Build history of the part. All positions in model axes, mm. A direction names the side the tool comes from. Give positions to 0.01 mm unless a question says otherwise; leave off trailing zeros. Order: outer loops, then holes, each group sorted by start corner. A loop starts at its lowest first (then second) coordinate and runs counter-clockwise, first axis right, second up. Notation, with made-up numbers: M 67.25,18.25 L 75.25,18.25 A19 cw 75.25,34.25 Z; hole C 30.5,45 d7. An arc over 180 degrees is marked long. One line per item, written item: value. Start each with the question number.
from build123d import *

# Parameters (mm, degrees)
SKETCH4_R           = 72
BOSS_EXTRUDE3_DEPTH = 5
SKETCH3_R           = 4
CUT_EXTRUDE6_DEPTH  = 102.946064171
SKETCH2_R           = 1.6
CUT_EXTRUDE1_DEPTH  = 102.946064171
GOPRO_DEPTH         = 102.946064171


with BuildPart() as part:
    # Sketch4 → Boss-Extrude3 (new body)
    with BuildSketch(Plane(origin=(0, 0, 0), x_dir=(0, 0, -1), z_dir=(1, 0, 0))):
        Circle(SKETCH4_R)
    extrude(amount=BOSS_EXTRUDE3_DEPTH)

    # Sketch3 → Cut-Extrude6 (cut, through all)
    with BuildSketch(Plane(origin=(0, 0, 0), x_dir=(0, 0, -1), z_dir=(1, 0, 0))):
        with Locations((47, 0)):
            Circle(SKETCH3_R)
        with Locations((-23.5, -40.703193978)):
            Circle(SKETCH3_R)
        with Locations((-23.5, 40.703193978)):
            Circle(SKETCH3_R)
    extrude(amount=CUT_EXTRUDE6_DEPTH, mode=Mode.SUBTRACT)

    # Sketch2 → Cut-Extrude1 (cut, through all)
    with BuildSketch(Plane(origin=(0, 0, 0), x_dir=(0, 0, -1), z_dir=(1, 0, 0))):
        with Locations((0, 66.5)):
            Circle(SKETCH2_R)
        with Locations((57.590689352, 33.25)):
            Circle(SKETCH2_R)
        with Locations((57.590689352, -33.25)):
            Circle(SKETCH2_R)
        with Locations((0, -66.5)):
            Circle(SKETCH2_R)
        with Locations((-57.590689352, -33.25)):
            Circle(SKETCH2_R)
        with Locations((-57.590689352, 33.25)):
            Circle(SKETCH2_R)
    extrude(amount=CUT_EXTRUDE1_DEPTH, mode=Mode.SUBTRACT)

    # Sketch1 → gopro (cut, through all)
    with BuildSketch(Plane(origin=(0, 0, 0), x_dir=(0, 0, -1), z_dir=(1, 0, 0))):
        with BuildLine():
            Line((-12, 15.5), (12, 15.5))
            ThreePointArc((12, 15.5), (14.828427125, 14.328427125), (16, 11.5))
            Line((16, 11.5), (16, -11.5))
            ThreePointArc((16, -11.5), (14.828427125, -14.328427125), (12, -15.5))
            Line((12, -15.5), (-12, -15.5))
            ThreePointArc((-12, -15.5), (-14.828427125, -14.328427125), (-16, -11.5))
            Line((-16, -11.5), (-16, 11.5))
            ThreePointArc((-16, 11.5), (-14.828427125, 14.328427125), (-12, 15.5))
        make_face()
    extrude(amount=GOPRO_DEPTH, mode=Mode.SUBTRACT)


solid = part.part
1) Drill centre lines: line 1 (Y direction, x = 2.85, z = 0); line 2 (Z direction, x = 2.5, y = -33.25); line 3 (Y direction, x = 1, z = -63). Where is each one in solid material? Low to high.
2) Slice it at B-B (z = 3.5). List the corners of the cut face in (x, y).
3) Pull direction Y, two halves, no side cores. Call faces 3 (the cylindrical face through (2.46, 32.64, 56.11)), 4 (the cylindrical face through (2.465, 14.297, 14.859)), 5 (the cylindrical face through (2.465, 71.387, 9.373)), 6 (the flat face through (5, 1, 17)): pulls with the +Y half, pulls with the -Y half, needs draft (parallel to the pull), parting line crosses it, or undercut.
4) Drop flat-ended pins along their axis: P1, Ø2, axis at x = 1.5, y = -41.5, coming from the +Z side; P2, Ø3, axis at y = 33.25, z = -57.59, coming from the -X side; P3, Ø3, axis at x = 0.5, z = 52, coming from the +Y side; P4, Ø2.5, axis at x = 3, y = 5.5, coming from the -Z side. Give the stop position or say it passes through.
5) Slice it at C-C (x = 3.1). State how many separate pieces and enclosed holes the cut face has, plus the area to 3 significant figures.
6) Slice it at D-D (z = 23.5). List the corners of the cut face in (x, y).
7) Tool access for faces 1 (the flat face through (2, 0, -16)), 2 (the flat face through (0, 1, 17)): list every direction of +Z, -Z, +X, -X, +Y, -Y with a clear straight run to the whole face (end or side of a thin tool).
8) Slice it at A-A (y = 0). List the corners of the cut face in (x, z).
Results list:
1. line 1: y = -72 to -68.1, -64.9 to -15.5, 15.5 to 64.9, 68.1 to 72
1. line 2: z = -63.86 to -59.19, -55.99 to 55.99, 59.19 to 63.86
1. line 3: y = -34.86 to 34.86
2. outline: M 0,-71.91 L 5,-71.91 L 5,-15.5 L 0,-15.5 Z; M 0,15.5 L 5,15.5 L 5,71.91 L 0,71.91 Z
3. face 3: undercut
3. face 4: undercut
3. face 5: parting line crosses it
3. face 6: needs draft
4. P1: stops at z = 59.53
4. P2: passes through
4. P3: stops at y = 51.32
4. P4: stops at z = -71.87
5. separate pieces: 1
5. enclosed holes: 10
5. area: 15,100 mm²
6. outline: M 0,-68.06 L 5,-68.06 L 5,-44.7 L 0,-44.7 Z; M 0,-36.7 L 5,-36.7 L 5,36.7 L 0,36.7 Z; M 0,44.7 L 5,44.7 L 5,68.06 L 0,68.06 Z
7. face 1: +X, -X
7. face 2: +Z, -Z, -X, +Y, -Y
8. outline: M 0,-72 L 5,-72 L 5,-51 L 0,-51 Z; M 0,-43 L 5,-43 L 5,-16 L 0,-16 Z; M 0,16 L 5,16 L 5,72 L 0,72 Z
